Autodesk Inventor part; units mm, degrees
ref_plane "YZ Plane" through (0, 0, 0) normal (1, 0, 0) x (0, 1, 0)
ref_plane "XZ Plane" through (0, 0, 0) normal (0, 1, 0) x (-1, 0, 0)
ref_plane "XY Plane" through (0, 0, 0) normal (0, 0, 1) x (1, 0, 0)
sketch "Sketch1" plane through (0, 0, 0) normal (0, 1, 0) x (-1, 0, 0)
  line L0 (-1.6252, -2.815) -> (-3.2505, 0)
  line L1 (-3.2505, 0) -> (-1.6252, 2.815)
  line L2 (-1.6252, 2.815) -> (1.6252, 2.815)
  line L3 (1.6252, 2.815) -> (3.2505, 0)
  line L4 (3.2505, 0) -> (1.6252, -2.815)
  line L5 (1.6252, -2.815) -> (-1.6252, -2.815)
  point P0 (0, 0)
  point P1 (0, 0)
  dimension "d0" = 5.63
extrude "Extrusion1" add sketch "Sketch1" along normal blind 9
sketch "Sketch2" plane through (0, 9, 0) normal (0, 1, 0) x (1, 0, 0)
  circle A0 centre (0, 0) radius 1.25
  dimension "d3" = 2.5
extrude "Extrusion2" add sketch "Sketch2" along normal blind 7
thread "Thread1"
chamfer "Chamfer1" distance 0.3 angle 45 1 edges at (-1.25, 16, 0)
sketch "Sketch3" plane through (-1.6252, 0, 2.815) normal (0, 0, 1) x (1, 0, 0)
  circle A0 centre (1.6252, 4.5) radius 1.25
  line L0 (0, 0) -> (3.2505, 0)
  point P0 (1.6252, 0)
  point P1 (1.6252, 0)
  dimension "d11" = 2.5
  dimension "d12" = 4.5
extrude "Extrusion3" cut sketch "Sketch3" against normal through all
sketch "Sketch4" plane through (0, 0, 0) normal (0, -1, 0) x (1, 0, 0)
  circle A0 centre (0, 0) radius 1.25
  dimension "d15" = 2.5
extrude "Extrusion4" cut sketch "Sketch4" against normal blind 4.5
properties part number "18102021-002-04" material "ABS Plastic"
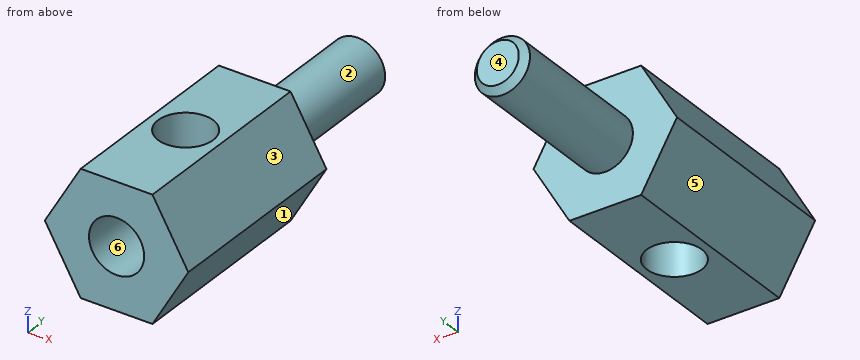
Source: CAD feature listing. Evaluate the final solid. Frame: model axes, mm. Face numbers are marked on the shaded views. A direction names the side the tool comes from. Round coordinates to 2 decimals unless told otherwise and drop trailing zeros. Order: outer loops, then holes, each group sorted by start corner. A loop starts at its lowest first (then second) coordinate and runs counter-clockwise, first axis right, second up. Notation, with made-up numbers: (24.25, 2.5) -> (47.25, 2.5) arc R33 cw to (47.25, 38.5) -> close; hole circle Ø9 at (-16.5, 14). An arc over 180 degrees is marked (long way). One line per item, written item: value. Start each with the question number.
Q1. Section query A-A (y = 8.75). Return the cut outline in (x, z) (1 decimal), plus the area to 3 significant figures.
Q2. Pin query (flat end, axial travel): pin 1 (3 mm diameter, centred on x = -1.5, z = 0, fed in from +Y); pin 2 (3 mm diameter, centred on y = 2.5, z = -2, fed in from -X); pin 3 (1.5 mm diameter, centred on x = -2, z = 2, fed in from +Y). Return the tip coordinate at first contact, or that it passes through.
Q3. Draft query along Z for the marked faces 3, 4, 5 and 6. Return one class per face: pulls with the +Z half, pulls with the -Z half, needs draft (parallel to the pull), parting line crosses it, or undercut.
Q4. Section query C-C (x = 0.25). Give the number of separate pieces and of enclosed holes in the cut face, plus the area to 3 significant figures.
Q5. Section query D-D (y = 11.5). Return the cut outline in (x, z).
Q6. Access query for the marked faces 1 and 2. Directions: +Z, -Z, +X, -X, +Y, -Y. A direction counts if a zero-diameter tool reaches every point of the face in a straight line with its end or side. Return the directions, or none.
Q7. Material intervals for probe 1 along Z at (x, y) = (0, 3) (3 decimals); probe 2 along Y at (x, z) = (0, 0.45); probe 3 along Y at (x, z) = (2, 1.75), sorted ascending.
Q8. Section query B-B (z = -2.3). Return the cut outline in (x, y).
Findings below:
1. outline: (-3.3, 0) -> (-1.6, -2.8) -> (1.6, -2.8) -> (3.3, 0) -> (1.6, 2.8) -> (-1.6, 2.8) -> close
1. area: 27.5 mm²
2. pin 1: y = 16
2. pin 2: x = -2.96
2. pin 3: y = 9
3. face 3: pulls with the +Z half
3. face 4: needs draft
3. face 5: pulls with the -Z half
3. face 6: undercut
4. separate pieces: 3
4. enclosed holes: 0
4. area: 45.9 mm²
5. outline: circle Ø2.5 at (0, 0)
6. face 1: -Z, +X, +Y, -Y
6. face 2: +Y
7. probe 1: -2.815 to -1.25, 1.25 to 2.815
7. probe 2: 5.75 to 16
7. probe 3: 0 to 9
8. outline: (-1.92, 0) -> (1.92, 0) -> (1.92, 9) -> (-1.92, 9) -> close; hole circle Ø2.5 at (0, 4.5)
